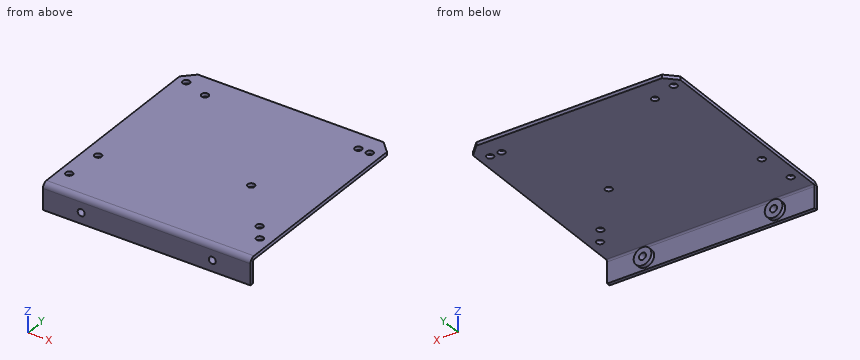
```python
from build123d import *

# Parameters (mm, degrees)
SM_BASE_FLANGE_2_DEPTH           = 1.6
SM_EDGE_FLANGE_2_STRIP_W         = 7.8732
SM_EDGE_FLANGE_2_STRIP_H         = 1.6
SM_EDGE_FLANGE_2_STRIP_CUT_DEPTH = 95
SM_EDGE_FLANGE_2_DEPTH           = 95
SKETCH_16_R                      = 4.05
EXTRUDE_1_DEPTH                  = 1.9
SKETCH_17_R                      = 1.6
CUT_EXTRUDE_1_DEPTH              = 106.203897266
SKETCH_18_R                      = 1.6
CUT_EXTRUDE_2_DEPTH              = 70.102966651


# Sheet-metal steps are written as plain solids
with BuildPart() as part:
    # 草图1 → 基体-法兰2 (new body)
    with BuildSketch(Plane.XY):
        Polygon((-47.5, 42.5), (-42.5, 47.5), (42.5, 47.5), (47.5, 42.5), (47.5, -47.5), (-47.5, -47.5), align=None)
    extrude(amount=-SM_BASE_FLANGE_2_DEPTH)

    # 边线-法兰2 strip (across the edge) → 边线-法兰2 strip cut (cut)
    with BuildSketch(Plane(origin=(47.5, -47.5, -1.6), x_dir=(0, 1, 0), z_dir=(-1, 0, 0))):
        with Locations((-3.2, -0.8)):
            Rectangle(SM_EDGE_FLANGE_2_STRIP_W, SM_EDGE_FLANGE_2_STRIP_H)
    extrude(amount=SM_EDGE_FLANGE_2_STRIP_CUT_DEPTH, mode=Mode.SUBTRACT)

    # 边线-法兰2 section (across the edge) → 边线-法兰2 (add)
    with BuildSketch(Plane(origin=(47.5, -47.5, -1.6), x_dir=(0, 1, 0), z_dir=(-1, 0, 0))):
        with BuildLine():
            Line((-1.6, 0.7366), (-1.6, 10.4))
            Line((-1.6, 10.4), (0, 10.4))
            Line((0, 10.4), (0, 0.7366))
            ThreePointArc((0, 0.7366), (0.215745145, 0.215745145), (0.7366, 0))
            Line((0.7366, 0), (0.7366, -1.6))
            ThreePointArc((0.7366, -1.6), (-0.915625705, -0.915625705), (-1.6, 0.7366))
        make_face()
    extrude(amount=SM_EDGE_FLANGE_2_DEPTH)

    # 草图16 → 凸台-拉伸1 (add)
    with BuildSketch(Plane(origin=(0, -47.5, 0), x_dir=(1, 0, 0), z_dir=(0, 1, 0))):
        with Locations(Location((-30, 7, 0), (0, 0, 90))):
            Circle(SKETCH_16_R)
    extrude_1 = extrude(amount=EXTRUDE_1_DEPTH)

    # 草图17 → 切除-拉伸1 (cut, through all)
    with BuildSketch(Plane(origin=(0, -45.6, 0), x_dir=(1, 0, 0), z_dir=(0, 1, 0))):
        with Locations(Location((-30, 7, 0), (0, 0, 270))):
            Circle(SKETCH_17_R)
    cut_extrude_1 = extrude(amount=-CUT_EXTRUDE_1_DEPTH, mode=Mode.SUBTRACT)

    # 镜向1: 凸台-拉伸1, 切除-拉伸1 across plane
    add(extrude_1.mirror(Plane(origin=(0, 0, 0), x_dir=(0, 0, 1), z_dir=(1, 0, 0))))
    add(cut_extrude_1.mirror(Plane(origin=(0, 0, 0), x_dir=(0, 0, 1), z_dir=(1, 0, 0))), mode=Mode.SUBTRACT)

    # 草图18 → 切除-拉伸2 (cut, through all)
    with BuildSketch(Plane(origin=(0, 0, -1.6), x_dir=(-1, 0, 0), z_dir=(0, 0, -1))):
        with Locations((-42.5, 38.3)):
            Circle(SKETCH_18_R)
        with Locations((32, 36.9)):
            Circle(SKETCH_18_R)
        with Locations((43.1, 40.6)):
            Circle(SKETCH_18_R)
        with Locations((-18.5, -6.1)):
            Circle(SKETCH_18_R)
        with Locations((-37.4, -28.2)):
            Circle(SKETCH_18_R)
        with Locations((-42.4, -35.3)):
            Circle(SKETCH_18_R)
        with Locations((41.3, -21.2)):
            Circle(SKETCH_18_R)
        with Locations((43.1, -37.9)):
            Circle(SKETCH_18_R)
        with Locations((-37.3, 38.3)):
            Circle(SKETCH_18_R)
    extrude(amount=-CUT_EXTRUDE_2_DEPTH, mode=Mode.SUBTRACT)


solid = part.part
```
Can you work these out from the model? Positions are in its coordinate system, mm. Give positions to 0.01 mm unless a question says otherwise; leave off trailing zeros. Write each loop counter-clockwise with the first axis right and the second up, starting at its lowest first coordinate (ties: lowest second). Pieces come first, ordered by that corner, then holes. Notation, with made-up numbers: (24, -11) -> (81, -11) arc R23 ccw to (81, 11) -> close; hole circle Ø2 at (-1.75, 50). An arc over 180 degrees is marked (long way). One line per item, written item: value.
Q1. For P1, Ø2.5, axis at x = 18.5, y = -6.1, coming from the +Z side; P2, Ø6.5, axis at x = 30, z = -7.5, coming from the +Y side; P3, Ø5, axis at x = 42.4, y = -35.3, coming from the -Z side; P4, Ø3, axis at x = -4.5, z = -6.5, coming from the +Y side, each with a flat end and sliding along its axis, tell me the tip position at first contact or that it passes through.
Results found:
P1: passes through
P2: stops at y = -45.6
P3: stops at z = -1.6
P4: stops at y = -47.5
Q2. Please list where these lines run through material, in increasing order: line 1 (Y direction, x = 42.4, z = -1); line 2 (Y direction, x = 42.4, z = -0.7); line 3 (Z direction, x = -5, y = -3). Write a range as [from, to].
Results found:
line 1: y = [-48.68, -36.9], [-33.7, 36.7], [39.9, 47.5]
line 2: y = [-48.43, -36.9], [-33.7, 36.7], [39.9, 47.5]
line 3: z = [-1.6, 0]
Q3. Imagine slicing it at B-B on y = -21.2. Please give me the cut outline in (x, z), and give its area (3 significant figures).
Results found:
outline: (-47.5, -1.6) -> (-42.9, -1.6) -> (-42.9, 0) -> (-47.5, 0) -> close; (-39.7, -1.6) -> (47.5, -1.6) -> (47.5, 0) -> (-39.7, 0) -> close
area: 147 mm^2
Q4. Imagine slicing it at C-C on x = 10.5. Please give me the cut outline in (y, z), and give its area (3 significant figures).
Results found:
outline: (-49.1, -12) -> (-47.5, -12) -> (-47.5, -2.34) arc R0.74 cw to (-46.76, -1.6) -> (47.5, -1.6) -> (47.5, 0) -> (-46.76, 0) arc R2.34 ccw to (-49.1, -2.34) -> close
area: 170 mm^2
Q5. Imagine slicing it at A-A on z = -7. Please give me the cut outline in (x, y), and give its area (3 significant figures).
Results found:
outline: (-47.5, -49.1) -> (-31.6, -49.1) -> (-31.6, -45.6) -> (-34.05, -45.6) -> (-34.05, -47.5) -> (-47.5, -47.5) -> close; (-28.4, -49.1) -> (28.4, -49.1) -> (28.4, -45.6) -> (25.95, -45.6) -> (25.95, -47.5) -> (-25.95, -47.5) -> (-25.95, -45.6) -> (-28.4, -45.6) -> close; (31.6, -49.1) -> (47.5, -49.1) -> (47.5, -47.5) -> (34.05, -47.5) -> (34.05, -45.6) -> (31.6, -45.6) -> close
area: 160 mm^2
